from build123d import *

# Parameters (mm, degrees)
SKETCH1_R           = 1
BOSS_EXTRUDE1_DEPTH = 10
SKETCH4_W           = 23
SKETCH4_H           = 7
CUT_EXTRUDE2_DEPTH  = 2


with BuildPart() as part:
    # Sketch1 → Boss-Extrude1 (new body)
    with BuildSketch(Plane.XY):
        Polygon((0, 0), (80, 0), (115.355339059, 35.355339059), (101.213203436, 49.497474683), (71.715728753, 20), (0, 20), align=None)
        with Locations((5, 10)):
            Circle(SKETCH1_R, mode=Mode.SUBTRACT)
    extrude(amount=BOSS_EXTRUDE1_DEPTH)

    # Sketch2 → Revolve2 (revolve)
    with BuildSketch(Plane.XY.offset(5)):
        with BuildLine():
            Line((108.284271247, 42.426406871), (142.163792523, 76.305928147))
            ThreePointArc((142.163792523, 76.305928147), (145.402623657, 44.93519468), (115.355339059, 35.355339059))
            Line((115.355339059, 35.355339059), (108.284271247, 42.426406871))
        make_face()
    revolve(axis=Axis((108.284271247, 42.426406871, 5), (0.7071067811865456, 0.7071067811865495, 0)))

    # Sketch4 → Cut-Extrude2 (cut)
    with BuildSketch(Plane(origin=(0, 0, 0), x_dir=(-1, 0, 0), z_dir=(0, 0, -1))):
        with Locations((-11.5, 10)):
            Rectangle(SKETCH4_W, SKETCH4_H)
    extrude(amount=-CUT_EXTRUDE2_DEPTH, mode=Mode.SUBTRACT)


solid = part.part
Design review of the part built by this model. Coordinates are the model's own, in mm. A direction names the side the tool comes from. Give positions to 0.01 mm unless a question says otherwise; leave off trailing zeros. Write each loop counter-clockwise with the first axis right and the second up, starting at its lowest first coordinate (ties: lowest second). Pieces come first, ordered by that corner, then holes. Notation, with made-up numbers: M 13,83 L 70,83 A19 ccw 70,87 Z; hole C 69,21.5 d2. An arc over 180 degrees is marked long. Answer as a JSON object with one key per item and string values. Group by question number.
1) We need section B-B (y = 16). Give the boundary of the cut face in (x, z), and give its area (3 significant figures).
2) We need section C-C (z = -11). Give the boundary of the cut face in (x, y), and give its area (3 significant figures).
3) We need section A-A (x = 13). Give the boundary of the cut face in (y, z), and give its area (3 significant figures).
4) Mouldability with a two-part tool opening along Y and no side actions: class faces 4 (the face through (108.2, 42.51, 11.91)), 5 (the face through (57, 14, 10)), 6 (the face through (12, 10, 2)) as released by +Y, released by -Y, zero draft, split by the parting line, or undercut.
5) Clearance check with flat-ended pins moving along their axes: pin 1 Ø3.5 at (x, y) = (9.5, 8.5) entering from -Z; pin 2 Ø1.5 at (x, z) = (73.5, 8.5) entering from +Y; pin 3 Ø1 at (y, z) = (36.5, 3.5) entering from +X. State where each tip first meets the part, or that it passes through.
6) Tool access review of faces 1 (the face through (39, 0, 5)), 2 (the face through (108.2, 42.51, -1.98)), 3 (the face through (36, 20, 5)): name each direction out of +Z, -Z, +X, -X, +Y, -Y from which nothing blocks a thin tool from reaching the whole face with its end or side.
7) We need section D-D (x = 42). Give the boundary of the cut face in (y, z).
8) For line 1 along Y through (x, z) = (5, 4); line 2 along X through (y, z) = (10, 5.25); line 3 along Z through (x, y) = (34.5, 5.5), list the stretches that pass through material, from the lowest coordinate up.
Answer key:
{
 "1": {"outline": "M 0,0 L 96,0 L 96,10 L 0,10 Z", "area": "960 mm²"},
 "2": {"outline": "C 124.49,58.63 d38.42", "area": "1,160 mm²"},
 "3": {"outline": "M 0,0 L 6.5,0 L 6.5,2 L 13.5,2 L 13.5,0 L 20,0 L 20,10 L 0,10 Z", "area": "186 mm²"},
 "4": {"face 4": "released by -Y", "face 5": "zero draft", "face 6": "undercut"},
 "5": {"pin 1": "stops at z = 2", "pin 2": "stops at y = 22.53", "pin 3": "stops at x = 136.94"},
 "6": {"face 1": "+Z, -Z, +X, -X, -Y", "face 2": "-Z, -X, -Y", "face 3": "+Z, -Z, -X, +Y"},
 "7": {"outline": "M 0,0 L 20,0 L 20,10 L 0,10 Z"},
 "8": {"line 1": "y = 0 to 9, 11 to 20", "line 2": "x = 0 to 4, 6 to 90", "line 3": "z = 0 to 10"}
}
